Geometry check sheet. Reference: the model listing, model coordinates, mm. Face numbers are marked on the shaded views. A direction names the side the tool comes from. Give positions to 0.01 mm unless a question says otherwise; leave off trailing zeros. Loops run counter-clockwise (first coordinate to the right, second up) from the corner with the lowest first, then second, coordinate; pieces in that order, holes last. Notation, with made-up numbers: (-9, 28) -> (19, 28) arc R29 ccw to (19, 60) -> close; hole circle Ø7 at (10.25, -25.5). An arc over 180 degrees is marked (long way). Answer as a JSON object with one key per item and string values.
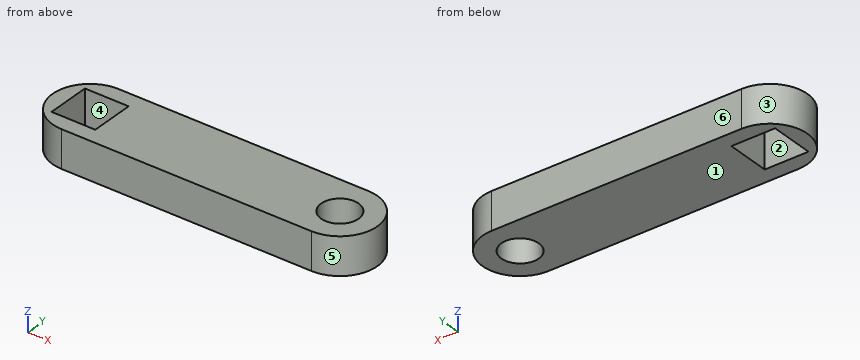
from build123d import *

# Parameters (mm, degrees)
ESQUISSE1_R        = 1.5
ESQUISSE1_W        = 3.5
ESQUISSE1_H        = 3.5
BOSS_EXTRU_1_DEPTH = 3


with BuildPart() as part:
    # Esquisse1 → Boss.-Extru.1 (new body)
    with BuildSketch(Plane.XY):
        with BuildLine():
            Line((0, 3), (20, 3))
            ThreePointArc((20, 3), (23, 0), (20, -3))
            Line((20, -3), (0, -3))
            ThreePointArc((0, -3), (-3, 0), (0, 3))
        make_face()
        with Locations((20, 0)):
            Circle(ESQUISSE1_R, mode=Mode.SUBTRACT)
        Rectangle(ESQUISSE1_W, ESQUISSE1_H, mode=Mode.SUBTRACT)
    extrude(amount=BOSS_EXTRU_1_DEPTH)


solid = part.part
1) Tool access check on the marked faces 1 and 2. Record the directions out of +Z, -Z, +X, -X, +Y, -Y that give a thin tool (end or side, any length) a straight path to the whole face; none if there is none.
Geometry check:
{"face 1": "-Z, +X, -X, +Y, -Y", "face 2": "+Z, -Z"}
2) Section check A-A on y = 0. Record the cut outline in (x, z).
Geometry check:
{"outline": "(-3, 0) -> (-1.75, 0) -> (-1.75, 3) -> (-3, 3) -> close; (1.75, 0) -> (18.5, 0) -> (18.5, 3) -> (1.75, 3) -> close; (21.5, 0) -> (23, 0) -> (23, 3) -> (21.5, 3) -> close"}
3) Material ranges on line 1 along X through (y, z) = (0.75, 2.25); line 2 along X through (y, z) = (0.1, 0.8); line 3 along Y through (x, z) = (20, 1.2), recorded low to high. Write a range as from..to.
Geometry check:
{"line 1": "x = -2.9..-1.75, 1.75..18.7, 21.3..22.9", "line 2": "x = -3..-1.75, 1.75..18.5, 21.5..23", "line 3": "y = -3..-1.5, 1.5..3"}
4) Section check B-B on z = 2.35. Record the cut outline in (x, y), plus the area to 3 significant figures.
Geometry check:
{"outline": "(0, -3) -> (20, -3) arc R3 ccw to (20, 3) -> (0, 3) arc R3 ccw to start; hole (-1.75, -1.75) -> (1.75, -1.75) -> (1.75, 1.75) -> (-1.75, 1.75) -> close; hole circle Ø3 at (20, 0)", "area": "129 mm2"}
5) Draft check along X on the marked faces 3, 4, 5 and 6. Enter one of: pulls with the +X half, pulls with the -X half, needs draft (parallel to the pull), parting line crosses it, or undercut.
Geometry check:
{"face 3": "pulls with the -X half", "face 4": "undercut", "face 5": "pulls with the +X half", "face 6": "needs draft"}
6) Section check D-D on y = -2.4. Record the cut outline in (x, z).
Geometry check:
{"outline": "(-1.8, 0) -> (21.8, 0) -> (21.8, 3) -> (-1.8, 3) -> close"}
7) Section check C-C on x = 19.5. Record the cut outline in (y, z).
Geometry check:
{"outline": "(-3, 0) -> (-1.41, 0) -> (-1.41, 3) -> (-3, 3) -> close; (1.41, 0) -> (3, 0) -> (3, 3) -> (1.41, 3) -> close"}
8) Depth check by flat-ended pin: P1, Ø1.5, axis at y = 2, z = 2.5, coming from the +X side; P2, Ø1.5, axis at x = -1, z = 2, coming from the -Y side. Enter the tip coordinate at first touch or a pass-through.
Geometry check:
{"P1": "stops at x = 22.73", "P2": "stops at y = -2.99"}
